Input: part model. Units: mm. Frame: model coordinates. A direction names the side the tool comes from. Round coordinates to 2 decimals unless told otherwise and drop trailing zeros. Loops run counter-clockwise (first coordinate to the right, second up) from the corner with the lowest first, then second, coordinate; pieces in that order, holes last. Notation, with made-up numbers: M 0,75 L 34,75 A16 cw 34,103 Z; hole C 23.5,83.5 d4. An arc over 180 degrees is marked long. Put each result on its own line as item: value. Start each with the question number.
1) Section B-B on x = 6.75. Output: boundary loops of the cut face in (y, z), plus the area to 3 significant figures.
2) Section A-A on y = 14. Output: boundary loops of the cut face in (x, z).
3) Reachability of faces 4 (the face through (7, 10, -3)), 5 (the face through (12, 14, -1)), 6 (the face through (2.5, 1.5, -10.3)) from +Z, -Z, +X, -X, +Y, -Y: full face, straight path, thin tool, end or side. Return the list, or none.
4) Line query: probe 1 along Y at (x, z) = (12.75, -18.5); probe 2 along Z at (x, y) = (1.5, 7.75); probe 3 along X at (y, z) = (12, -2.5). Output: solid intervals per line, ascending.
5) Section D-D on z = -1.5. Output: boundary loops of the cut face in (x, y).
6) Pin query (flat end, axial travel): pin 1 (7 mm diameter, centred on x = 6.5, y = 8, fed in from -Z); pin 2 (4.5 mm diameter, centred on x = 10, z = -10.5, fed in from +Y). Return the tip coordinate at first contact, or that it passes through.
7) Draft query along Y for faces 1 (the face through (7, 11.25, -1)), 2 (the face through (7, 1, -12.95)), 3 (the face through (7, 0, -6)). Return one class per face: +Y half, -Y half, draft (parallel to the pull), parting line (faces both ways), or undercut.
8) Section C-C on z = -10.2. Output: boundary loops of the cut face in (x, y).
from build123d import *

# Parameters (mm, degrees)
BOSS_EXTRUDE1_DEPTH = 14.5
CUT_EXTRUDE1_DEPTH  = 21
CUT_EXTRUDE2_DEPTH  = 21


with BuildPart() as part:
    # Sketch1 → Boss-Extrude1 (new body)
    with BuildSketch(Plane(origin=(0, 0, 0), x_dir=(0, 0, -1), z_dir=(1, 0, 0))):
        Polygon((0, 0), (0, 20), (3, 20), (3, 3), (20, 3), (20, 0), align=None)
    extrude(amount=BOSS_EXTRUDE1_DEPTH)

    # Sketch2 → Cut-Extrude1 (cut, through all)
    with BuildSketch(Plane.XY):
        with BuildLine():
            Line((5.25, 16.75), (9.25, 16.75))
            ThreePointArc((9.25, 16.75), (12, 14), (9.25, 11.25))
            Line((9.25, 11.25), (5.25, 11.25))
            ThreePointArc((5.25, 11.25), (2.5, 14), (5.25, 16.75))
        make_face()
    extrude(amount=-CUT_EXTRUDE1_DEPTH, mode=Mode.SUBTRACT)

    # Sketch3 → Cut-Extrude2 (cut, through all)
    with BuildSketch(Plane.XZ):
        with BuildLine():
            Line((5.25, -7.45), (9.25, -7.45))
            ThreePointArc((9.25, -7.45), (12, -10.2), (9.25, -12.95))
            Line((9.25, -12.95), (5.25, -12.95))
            ThreePointArc((5.25, -12.95), (2.5, -10.2), (5.25, -7.45))
        make_face()
    extrude(amount=-CUT_EXTRUDE2_DEPTH, mode=Mode.SUBTRACT)


solid = part.part
Geometry results:
1. outline: M 0,-20 L 3,-20 L 3,-12.95 L 0,-12.95 Z; M 0,-7.45 L 3,-7.45 L 3,-3 L 11.25,-3 L 11.25,0 L 0,0 Z; M 16.75,-3 L 20,-3 L 20,0 L 16.75,0 Z
1. area: 78.0 mm²
2. outline: M 0,-3 L 2.5,-3 L 2.5,0 L 0,0 Z; M 12,-3 L 14.5,-3 L 14.5,0 L 12,0 Z
3. face 4: -Z, +X, -X, +Y
3. face 5: +Z, -Z
3. face 6: +Y, -Y
4. probe 1: y = 0 to 3
4. probe 2: z = -3 to 0
4. probe 3: x = 0 to 3.36, 11.14 to 14.5
5. outline: M 0,0 L 14.5,0 L 14.5,20 L 0,20 Z; hole M 5.25,11.25 L 9.25,11.25 A2.75 ccw 9.25,16.75 L 5.25,16.75 A2.75 ccw Z
6. pin 1: stops at z = -3
6. pin 2: stops at y = 3
7. face 1: undercut
7. face 2: draft
7. face 3: -Y half
8. outline: M 0,0 L 2.5,0 L 2.5,3 L 0,3 Z; M 12,0 L 14.5,0 L 14.5,3 L 12,3 Z
